Part print with two shaded views. Sizes in mm from the minimum x, y, z corner. A direction names the side the tool comes from. Round coordinates to 2 decimals unless told otherwise and drop trailing zeros. Order: outer loops, then holes, each group sorted by start corner. A loop starts at its lowest first (then second) coordinate and runs counter-clockwise, first axis right, second up. Notation, with made-up numbers: (89, 11) - (148, 11) arc R21 cw to (148, 35) - close; hole circle Ø7 at (74.5, 3). An arc over 180 degrees is marked (long way). Use one line per item in the form item = value.
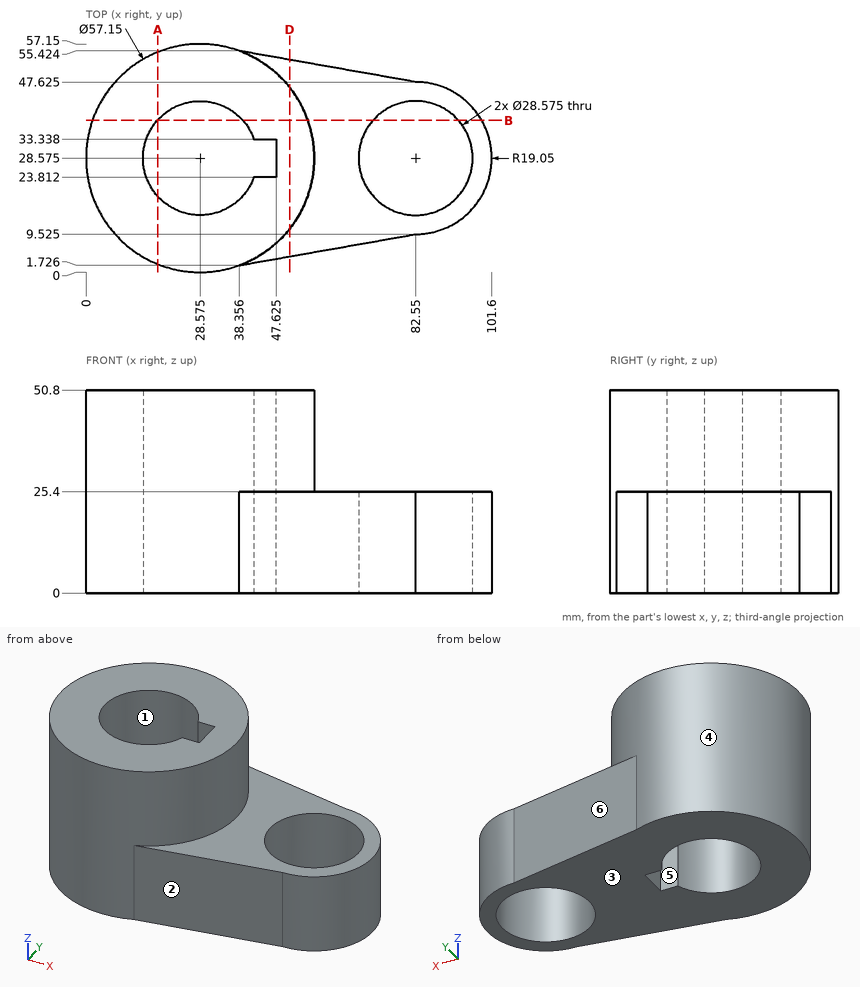
(1) Slice it at A-A on x = 18. Give the cut face in (y, z), then the cut area to 3 significant figures.
Report:
outline = (2.03, 0) - (18.97, 0) - (18.97, 50.8) - (2.03, 50.8) - close; (38.18, 0) - (55.12, 0) - (55.12, 50.8) - (38.18, 50.8) - close
area = 1,720 mm2
(2) Tool access for the marked faces 4, 5 and 6: list every direction of +Z, -Z, +X, -X, +Y, -Y with a clear straight run to the whole face (end or side of a thin tool).
Report:
face_4 = +Z
face_5 = +Z, -Z
face_6 = +Z, -Z, +X, +Y
(3) Slice it at D-D on x = 51. Give the cut face in (y, z) (1 decimal).
Report:
outline = (4, 0) - (53.2, 0) - (53.2, 25.4) - (46.3, 25.4) - (46.3, 50.8) - (10.9, 50.8) - (10.9, 25.4) - (4, 25.4) - close
(4) Probe probe 1 along X at (y, z) = (29.5, 10) (1 decimal); probe 2 along X at (y, z) = (32, 9.5) (1 decimal); probe 3 along Y at (x, z) = (28.5, 31). List the from-to ranges inside material, lowest first. Write a range as [from, to].
Report:
probe_1 = [0, 14.3], [47.6, 68.3], [96.8, 101.6]
probe_2 = [0.2, 14.7], [47.6, 68.7], [96.4, 101.3]
probe_3 = [0, 14.29], [42.86, 57.15]
(5) Pin check, flat tips, straight feed: pin 1 (10 mm diameter, centred on y = 43, z = 45, fed in from -X); pin 2 (6 mm diameter, centred on x = 46, z = 18.5, fed in from +Y) (1 decimal); pin 3 (10 mm diameter, centred on y = 44, z = 40.5, fed in from +X). Stop position of each tip, or through.
Report:
pin_1 = 1.6
pin_2 = 54.6
pin_3 = 55.18
(6) Slice it at B-B on y = 38. Count the separate pieces of the cut face and the enclosed holes in it, then the cut area to 3 significant figures.
Report:
separate_pieces = 3
enclosed_holes = 0
area = 2,210 mm2
(7) Pull direction Y, two halves, no side cores. Call the marked faces 1, 2 and 3: released by +Y, released by -Y, zero draft, split by the parting line, or undercut.
Report:
face_1 = undercut
face_2 = released by -Y
face_3 = zero draft
